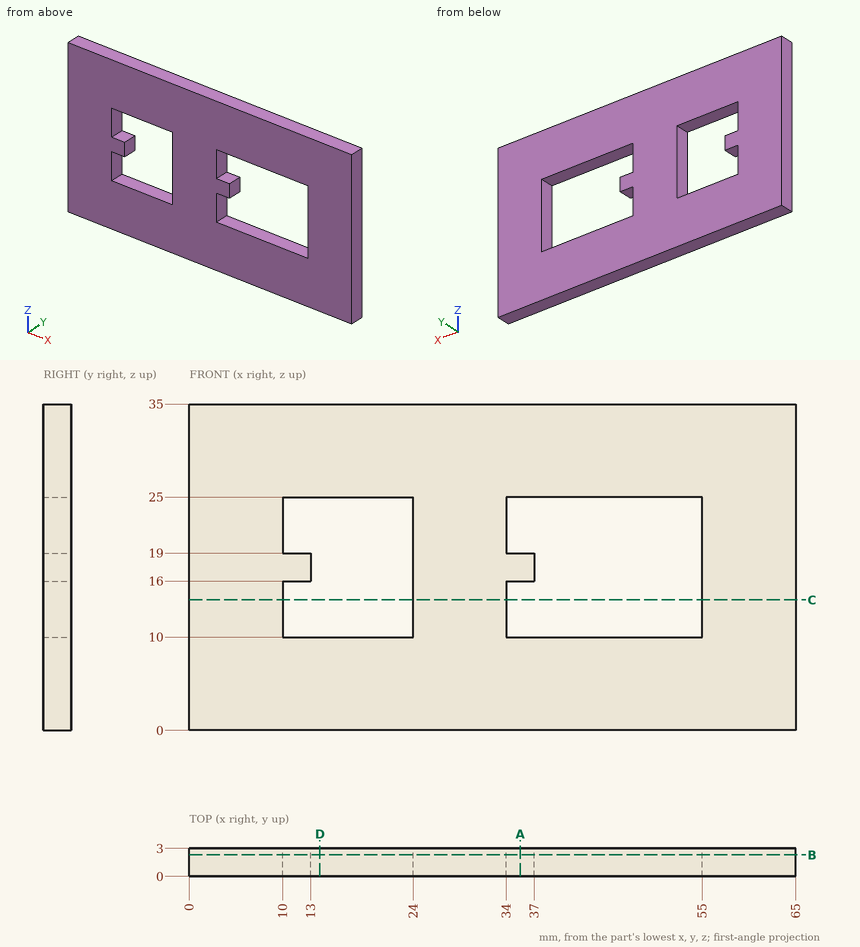
Could you check a few things on this drawing? It's one solid part, dimensions in mm from its lowest x, y, z. Give positions to 0.01 mm unless a question says otherwise; leave off trailing zeros. Loops run counter-clockwise (first coordinate to the right, second up) from the corner with the lowest first, then second, coordinate; pieces in that order, holes last. Notation, with made-up numbers: M 25.25,65 L 55.25,65 A15 cw 55.25,71 Z; hole C 26.25,38 d1. An arc over 180 degrees is marked long. One line per question, with ' | ' between items. Start each with the question number.
Q1. If we section it at D-D (x = 14): Please give me the cut outline in (y, z), plus the area to 3 significant figures.
Q2. If we section it at C-C (z = 14): Please give me the cut outline in (x, y).
Q3. If I drill on line 1 (Z direction, x = 36, y = 1.6); line 2 (X direction, y = 2.1, z = 14.5); line 3 (Z direction, x = 18.5, y = 1.65), over which ranges is the centre line in solid material (lowest first)? Write a range as from..to.
Q4. If we section it at A-A (x = 35.5): Please give me the cut outline in (y, z).
Q5. If we section it at B-B (y = 2.3): Please give me the cut outline in (x, z).
Computed:
1) outline: M 0,0 L 3,0 L 3,10 L 0,10 Z; M 0,25 L 3,25 L 3,35 L 0,35 Z | area: 60.0 mm²
2) outline: M 0,0 L 10,0 L 10,3 L 0,3 Z; M 24,0 L 34,0 L 34,3 L 24,3 Z; M 55,0 L 65,0 L 65,3 L 55,3 Z
3) line 1: z = 0..10, 16..19, 25..35 | line 2: x = 0..10, 24..34, 55..65 | line 3: z = 0..10, 25..35
4) outline: M 0,0 L 3,0 L 3,10 L 0,10 Z; M 0,16 L 3,16 L 3,19 L 0,19 Z; M 0,25 L 3,25 L 3,35 L 0,35 Z
5) outline: M 0,0 L 65,0 L 65,35 L 0,35 Z; hole M 10,10 L 24,10 L 24,25 L 10,25 L 10,19 L 13,19 L 13,16 L 10,16 Z; hole M 34,10 L 55,10 L 55,25 L 34,25 L 34,19 L 37,19 L 37,16 L 34,16 Z
